Autodesk Inventor part; units mm, degrees
ref_plane "YZ Plane" through (0, 0, 0) normal (1, 0, 0) x (0, 1, 0)
ref_plane "XZ Plane" through (0, 0, 0) normal (0, 1, 0) x (-1, 0, 0)
ref_plane "XY Plane" through (0, 0, 0) normal (0, 0, 1) x (1, 0, 0)
sketch "Sketch1" plane through (0, 0, 0) normal (0, 0, 1) x (1, 0, 0)
  line L0 (-8, 10) -> (8, 10)
  line L1 (10, 8) -> (10, -8)
  line L2 (8, -10) -> (-8, -10)
  line L3 (-10, -8) -> (-10, 8)
  line L4 (0, 0) -> (10, 0) construction
  line L5 (0, 0) -> (0, 10) construction
  arc A0 (-8, 10) -> (-10, 8) centre (-8, 8) ccw
  arc A1 (-10, -8) -> (-8, -10) centre (-8, -8) ccw
  arc A2 (8, -10) -> (10, -8) centre (8, -8) ccw
  arc A3 (10, 8) -> (8, 10) centre (8, 8) ccw
  point P0 (10, -10)
  point P1 (10, 10)
  dimension "d1" = 20
  dimension "d3" = 16
extrude "Extrusion1" add sketch "Sketch1" along normal blind 33
sketch "Sketch2" plane through (0, 0, 33) normal (0, 0, 1) x (1, 0, 0)
  circle A0 centre (0, 0) radius 7.5
  dimension "d6" = 15
extrude "Extrusion2" add sketch "Sketch2" along normal blind 1.7
sketch "Sketch3" plane through (0, 0, 34.7) normal (0, 0, 1) x (1, 0, 0)
  circle A0 centre (0, 0) radius 2
  dimension "d9" = 4
extrude "Extrusion3" add sketch "Sketch3" along normal blind 10 from surface at -1.7
sketch "Sketch4" plane through (-8, -10, 0) normal (0, -1, 0) x (1, 0, 0)
  line L0 (16, 0) -> (0, 0)
  line L1 (2, 0) -> (14, 0)
  line L2 (14, 0) -> (14, 8)
  line L3 (8, 8) -> (2, 8)
  line L4 (2, 8) -> (2, 0)
  line L5 (8, 0) -> (8, 46.0613) construction
  line L6 (8, 8) -> (14, 8)
  dimension "d12" = 12
  dimension "d13" = 8
extrude "Extrusion4" add sketch "Sketch4" along normal blind 1.75
sketch "Sketch5" plane through (0, 0, 33) normal (0, 0, 1) x (1, 0, 0)
  line L0 (8, 10) -> (-8, 10) construction
  line L1 (6, -10) -> (8, -10) construction
  line L2 (-8, 10) -> (8, 10) construction
  line L3 (8, 10) -> (8, -10) construction
  line L4 (8, -10) -> (-8, -10) construction
  line L5 (-8, -10) -> (-8, 10) construction
  line L6 (10, -8) -> (10, 8) construction
  line L7 (-10, 8) -> (-10, -8) construction
  line L8 (10, 8) -> (-10, 8) construction
  line L9 (-10, 8) -> (-10, -8) construction
  line L10 (-10, -8) -> (10, -8) construction
  line L11 (10, -8) -> (10, 8) construction
  point P0 (0, 0)
  point P1 (-8, 8)
  point P2 (8, 8)
  point P3 (8, -8)
  point P4 (-8, -8)
hole "Hole1" at (-8, 8, 33) at (8, 8, 33) at (8, -8, 33) at (-8, -8, 33) direction (0, 0, -1) diameter 1.567 depth 8
sketch "Sketch6" plane through (0, 0, 0) normal (0, 0, -1) x (-1, 0, 0)
  line L0 (-4, -10.25) -> (4, -10.25)
  line L1 (4, -10.25) -> (4, -10.75)
  line L2 (-4, -10.75) -> (-4, -10.25)
  line L3 (0, 0) -> (0, -11.75) construction
  line L4 (-6, -11.75) -> (6, -11.75) construction
  line L5 (4, -10.75) -> (0, -10.75)
  line L6 (-4, -10.75) -> (0, -10.75)
  line L7 (8, -10) -> (-8, -10)
  dimension "d23" = 8
  dimension "d24" = 0.5
  dimension "d25" = 1
extrude "Extrusion5" [suppressed]
equation "\"d13\" = extrusionHeight"
equation "\"d21\" = screwDepth"
equation "\"d23\" = ribbonWidth"
equation "\"d24\" = ribbonThickness"
equation "\"d25\" = ribbonEdgeOffset"
equation "\"extrusionHeight\" = 8"
equation "\"screwDepth\" = 8"
equation "\"ribbonWidth\" = 8"
equation "\"ribbonThickness\" = 0.5"
equation "\"ribbonEdgeOffset\" = 1"
properties part number "StepperMotor"
Can you work these out from the model? Positions are in its coordinate system, mm. A direction names the side the tool comes from. Round coordinates to 2 decimals unless told otherwise and drop trailing zeros. Order: outer loops, then holes, each group sorted by start corner. A loop starts at its lowest first (then second) coordinate and runs counter-clockwise, first axis right, second up.
(1) If we section it at C-C (x = 0): Please give me the cut outline in (y, z), plus the area to 3 significant figures.
Results are:
outline: (-11.75, 0) - (10, 0) - (10, 33) - (7.5, 33) - (7.5, 34.7) - (2, 34.7) - (2, 43) - (-2, 43) - (-2, 34.7) - (-7.5, 34.7) - (-7.5, 33) - (-10, 33) - (-10, 8) - (-11.75, 8) - close
area: 733 mm2
(2) We'd pull the mould along X, two halves only. Please class faces 1 (the face through (0, -11.75, 4)), 2 (the face through (-7.493, -0.33, 33.838)), 3 (the face through (-8, -8, 25)): +X half, -X half, draft (parallel to the pull), parting line (faces both ways), or undercut.
Results are:
face 1: draft
face 2: parting line
face 3: undercut
(3) I'm going to push flat-ended pins straight in: pin 1 (0.8 mm diameter, centred on x = -8, y = -8, fed in from +Z); pin 2 (1.9 mm diameter, centred on x = 2, y = -10.5, fed in from +Z); pin 3 (8 mm diameter, centred on x = -1.5, z = 19.5, fed in from -Y). Where does each tip first touch, or does it pass through?
Results are:
pin 1: stops at z = 25
pin 2: stops at z = 33
pin 3: stops at y = -10
(4) If we section it at D-D (z = 12): Please give me the cut outline in (x, y), plus the area to 3 significant figures.
Results are:
outline: (-10, -8) arc R2 ccw to (-8, -10) - (8, -10) arc R2 ccw to (10, -8) - (10, 8) arc R2 ccw to (8, 10) - (-8, 10) arc R2 ccw to (-10, 8) - close
area: 397 mm2
(5) If we section it at A-A (y = 0): Please give me the cut outline in (x, z).
Results are:
outline: (-10, 0) - (10, 0) - (10, 33) - (7.5, 33) - (7.5, 34.7) - (2, 34.7) - (2, 43) - (-2, 43) - (-2, 34.7) - (-7.5, 34.7) - (-7.5, 33) - (-10, 33) - close
(6) If I drill on L1, parallel to Y at x = 8, z = 28.75; L2, parallel to Z at x = 7.5, y = -6.25, over which ranges is the centre line in solid material (lowest first)?
Results are:
L1: y = -10 to -8.78, -7.22 to 7.22, 8.78 to 10
L2: z = 0 to 33
(7) On a 3-axis mill with a long thin cutter (end or side, diameter ignored), from which of +Z, -Z, +X, -X, +Y, -Y can I reach the whole of each face in a straight line? I mean faces 4 (the face through (0, -11, 8)), 5 (the face through (8, -8, 25)), 6 (the face through (9.43, -9.4, 16.27)). Say none if no direction works.
Results are:
face 4: +Z, +X, -X, -Y
face 5: +Z
face 6: +Z, -Z, +X, -Y
(8) If we section it at B-B (z = 30): Please give me the cut outline in (x, y).
Results are:
outline: (-10, -8) arc R2 ccw to (-8, -10) - (8, -10) arc R2 ccw to (10, -8) - (10, 8) arc R2 ccw to (8, 10) - (-8, 10) arc R2 ccw to (-10, 8) - close; hole circle Ø1.57 at (-8, -8); hole circle Ø1.57 at (-8, 8); hole circle Ø1.57 at (8, -8); hole circle Ø1.57 at (8, 8)
